Here's how the part is built. I have some questions about the finished solid (model axes, mm). Face numbers are marked on the shaded views. A direction names the side the tool comes from. Coordinates: 2 decimals unless noted, no trailing zeros. Write each loop counter-clockwise with the first axis right and the second up, starting at its lowest first coordinate (ties: lowest second). Pieces come first, ordered by that corner, then holes. Notation, with made-up numbers: (14, -35) -> (38, -35) arc R16 cw to (38, -21) -> close; hole circle Ø1 at (60, -21). An arc over 180 degrees is marked (long way). Use a Markdown table: item, result. Add a question column.
Item 1: If I drill on line 1 along Y through (x, z) = (3, 1.95); line 2 along Y through (x, z) = (1.5, 2.1); line 3 along Z through (x, y) = (-2, 3), over which ranges is the centre line in solid material (lowest first)? Write a range as from..to.
Item 2: Imagine slicing it at B-B, the plane x = 5.5. Write out the boundary of the cut face in (y, z), and give its area (3 significant figures).
Item 3: Imagine slicing it at A-A, the plane z = -1.2. Write out the boundary of the cut face in (x, y), and give its area (3 significant figures).
Item 4: On a 3-axis mill with a long thin cutter (end or side, diameter ignored), from which of +Z, -Z, +X, -X, +Y, -Y can I reach the whole of each face in a straight line? I mean the marked faces 1, 2 and 3. Say none if no direction works.
Item 5: Will these pins go through, and if not, where does the flat tip stop? pin 1 Ø0.6 at (x, z) = (4, 2) entering from +Y; pin 2 Ø2 at (y, z) = (-12.5, -1.5) entering from +X.
Autodesk Inventor part; units mm, degrees
ref_plane "YZ Plane" through (0, 0, 0) normal (1, 0, 0) x (0, 1, 0)
ref_plane "XZ Plane" through (0, 0, 0) normal (0, 1, 0) x (-1, 0, 0)
ref_plane "XY Plane" through (0, 0, 0) normal (0, 0, 1) x (1, 0, 0)
sketch "스케치1" plane through (0, 0, 0) normal (0, 0, 1) x (1, 0, 0)
  line L0 (-6, 13) -> (6, 13)
  line L1 (6, 13) -> (6, -13)
  line L2 (6, -13) -> (-6, -13)
  line L3 (-6, -13) -> (-6, 13)
  line L4 (-6, 13) -> (6, -13) construction
  line L5 (6, 13) -> (-6, -13) construction
  point P0 (0, 0)
  dimension "d0" = 12
  dimension "d1" = 26
extrude "돌출1" add sketch "스케치1" along normal mid plane 5
fillet "모깎기1" radius 3 4 edges at (6, 13, 0) (-6, 13, 0) (6, -13, 0) (-6, -13, 0)
sketch "스케치2" plane through (-3, 13, 2.5) normal (0, 1, 0) x (1, 0, 0)
  circle A0 centre (3, 2.5) radius 2
  dimension "d5" = 4
extrude "돌출2" add sketch "스케치2" along normal blind 4.5 and the other way blind 30.5
sketch "스케치3" plane through (0, 0, 2.5) normal (0, 0, 1) x (1, 0, 0)
  line L0 (-4.5251, 3.4564) -> (4.6298, 3.4564) construction
  line L1 (4.6298, 3.4564) -> (4.6298, -2.8858) construction
  line L2 (4.6298, -2.8858) -> (-4.5251, -2.8858) construction
  line L3 (-4.5251, -2.8858) -> (-4.5251, 3.4564) construction
  spline S0 degree 2 poles (-4.2483, 1.3506) (-4.2483, 1.8202) (-3.9418, 2.6012) (-3.6749, 2.883) knots 0 0 0 1 2 2 2
  spline S1 degree 2 poles (-3.6749, 2.883) (-3.4228, 3.1549) (-2.6863, 3.4564) (-2.3106, 3.4564) knots 0 0 0 1 2 2 2
  spline S2 degree 2 poles (-2.3106, 3.4564) (-1.8904, 3.4564) (-1.2082, 3.1746) (-0.9561, 2.9077) knots 0 0 0 1 2 2 2
  spline S3 degree 2 poles (-0.9561, 2.9077) (-0.6397, 2.5715) (-0.2937, 1.484) (-0.2937, 0.6486) knots 0 0 0 1 2 2 2
  spline S4 degree 2 poles (-0.2937, 0.6486) (-0.2937, -0.1077) (-0.6348, -1.4622) (-0.966, -1.912) knots 0 0 0 1 2 2 2
  spline S5 degree 2 poles (-0.966, -1.912) (-1.317, -2.3866) (-2.3056, -2.8858) (-3.0273, -2.8858) knots 0 0 0 1 2 2 2
  spline S6 degree 2 poles (-3.0273, -2.8858) (-3.1905, -2.8858) (-3.5612, -2.8512) (-3.7194, -2.8018) knots 0 0 0 1 2 2 2
  line L4 (-3.7194, -2.8018) -> (-3.7194, -2.0158)
  line L5 (-3.7194, -2.0158) -> (-3.6798, -2.0158)
  spline S7 degree 2 poles (-3.6798, -2.0158) (-3.576, -2.0751) (-3.141, -2.1789) (-2.9186, -2.1789) knots 0 0 0 1 2 2 2
  spline S8 degree 2 poles (-2.9186, -2.1789) (-2.1178, -2.1789) (-1.2033, -1.1211) (-1.139, -0.1423) knots 0 0 0 1 2 2 2
  spline S9 degree 2 poles (-1.139, -0.1423) (-1.4653, -0.3648) (-2.0585, -0.5674) (-2.4094, -0.5674) knots 0 0 0 1 2 2 2
  spline S10 degree 2 poles (-2.4094, -0.5674) (-2.7456, -0.5674) (-3.3042, -0.4191) (-3.5859, -0.2066) knots 0 0 0 1 2 2 2
  spline S11 degree 2 poles (-3.5859, -0.2066) (-3.9122, 0.0455) (-4.2483, 0.8117) (-4.2483, 1.3506) knots 0 0 0 1 2 2 2
  spline S12 degree 2 poles (-1.1192, 0.8315) (-1.1192, 1.4494) (-1.3466, 2.2305) (-1.5493, 2.443) knots 0 0 0 1 2 2 2
  spline S13 degree 2 poles (-1.5493, 2.443) (-1.7273, 2.6408) (-2.098, 2.7891) (-2.3155, 2.7891) knots 0 0 0 1 2 2 2
  spline S14 degree 2 poles (-2.3155, 2.7891) (-2.8197, 2.7891) (-3.4179, 2.0673) (-3.4179, 1.3852) knots 0 0 0 1 2 2 2
  spline S15 degree 2 poles (-3.4179, 1.3852) (-3.4179, 0.9996) (-3.2201, 0.5003) (-3.0026, 0.3224) knots 0 0 0 1 2 2 2
  spline S16 degree 2 poles (-3.0026, 0.3224) (-2.8444, 0.1938) (-2.4539, 0.1098) (-2.2265, 0.1098) knots 0 0 0 1 2 2 2
  spline S17 degree 2 poles (-2.2265, 0.1098) (-1.9645, 0.1098) (-1.3615, 0.2927) (-1.1341, 0.4459) knots 0 0 0 1 2 2 2
  spline S18 degree 2 poles (-1.1341, 0.4459) (-1.1291, 0.5053) (-1.1192, 0.7079) (-1.1192, 0.8315) knots 0 0 0 1 2 2 2
  line L6 (4.4222, -0.6712) -> (3.6955, -0.6712)
  line L7 (3.6955, -0.6712) -> (3.6955, -2.7672)
  line L8 (3.6955, -2.7672) -> (2.9095, -2.7672)
  line L9 (2.9095, -2.7672) -> (2.9095, -0.6712)
  line L10 (2.9095, -0.6712) -> (0.2155, -0.6712)
  line L11 (0.2155, -0.6712) -> (0.2155, 0.1889)
  line L12 (0.2155, 0.1889) -> (2.9441, 3.3328)
  line L13 (2.9441, 3.3328) -> (3.6955, 3.3328)
  line L14 (3.6955, 3.3328) -> (3.6955, -0.0138)
  line L15 (3.6955, -0.0138) -> (4.4222, -0.0138)
  line L16 (4.4222, -0.0138) -> (4.4222, -0.6712)
  line L17 (2.9095, -0.0138) -> (2.9095, 2.3689)
  line L18 (2.9095, 2.3689) -> (0.8581, -0.0138)
  line L19 (0.8581, -0.0138) -> (2.9095, -0.0138)
  point P0 (0, 0)
extrude "돌출3" cut sketch "스케치3" against normal blind 1
properties part number "16-2"
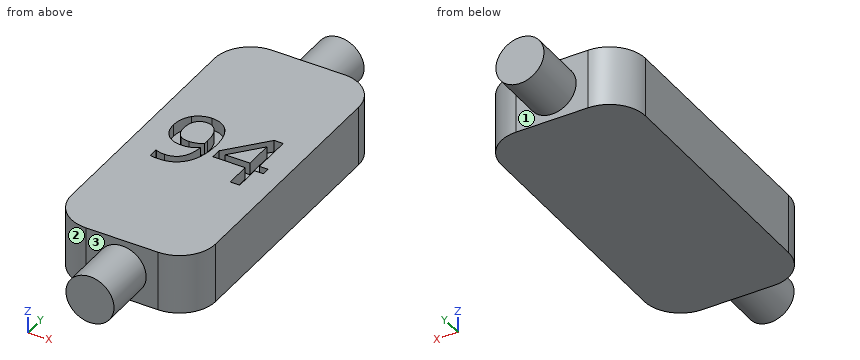
Ans:
| question | item | result |
|---|---|---|
| 1 | line 1 | y = -13..-2.77, 3.33..13 |
| 1 | line 2 | y = -13..-0.67, -0.01..0.73, 1.67..13 |
| 1 | line 3 | z = -2.5..1.5 |
| 2 | outline | (-11.66, -2.5) -> (11.66, -2.5) -> (11.66, 2.5) -> (-11.66, 2.5) -> close |
| 2 | area | 117 mm^2 |
| 3 | outline | (-6, -10) arc R3 ccw to (-3, -13) -> (-1.6, -13) -> (-1.6, -17.5) -> (1.6, -17.5) -> (1.6, -13) -> (3, -13) arc R3 ccw to (6, -10) -> (6, 10) arc R3 ccw to (3, 13) -> (1.6, 13) -> (1.6, 17.5) -> (-1.6, 17.5) -> (-1.6, 13) -> (-3, 13) arc R3 ccw to (-6, 10) -> close |
| 3 | area | 333 mm^2 |
| 4 | face 1 | +Y |
| 4 | face 2 | +Z, -Z, -X, -Y |
| 4 | face 3 | -Y |
| 5 | pin 1 | stops at y = 12.92 |
| 5 | pin 2 | stops at x = 5.6 |
